```python
from build123d import *

# Parameters (mm, degrees)
ESBO_O1_R                = 1.5
RESSALTO_EXTRUS_O1_DEPTH = 2
ESBO_O2_R                = 1.5
RESSALTO_EXTRUS_O2_DEPTH = 1
ESBO_O4_R                = 2.5
ESBO_O4_R_2              = 1.5
RESSALTO_EXTRUS_O3_DEPTH = 2
ESBO_O5_R                = 1.5
RESSALTO_EXTRUS_O4_DEPTH = 2
ESBO_O6_R                = 1.648621548
RESSALTO_EXTRUS_O5_DEPTH = 1
ESBO_O7_W                = 11.938868243
ESBO_O7_H                = 15.738508052
CORTE_EXTRUS_O1_DEPTH    = 6
RESSALTO_EXTRUS_O6_START = -2
ESBO_O8_R                = 2.148621548
RESSALTO_EXTRUS_O6_DEPTH = 0.5
RESSALTO_EXTRUS_O7_START = -2.5
ESBO_O9_R                = 2.148621548
RESSALTO_EXTRUS_O7_DEPTH = 0.5
RESSALTO_EXTRUS_O8_START = -2.5
ESBO_O10_R               = 2
RESSALTO_EXTRUS_O8_DEPTH = 0.5
RESSALTO_EXTRUS_O9_START = -2
ESBO_O11_R               = 2
RESSALTO_EXTRUS_O9_DEPTH = 0.5


with BuildPart() as part:
    # Esboço1 → Ressalto-extrusão1 (new body)
    with BuildSketch(Plane.XY):
        with BuildLine():
            Line((-1.198777863, 9.438372785), (-2.475695902, 0.347749621))
            ThreePointArc((-2.475695902, 0.347749621), (-1.4263e-05, -2.5), (2.47569987, 0.347721373))
            Line((2.47569987, 0.347721373), (1.198866989, 9.438491296))
            ThreePointArc((1.198866989, 9.438491296), (-7.4142e-05, 11.839999998), (-1.198777863, 9.438372785))
        make_face()
        Circle(ESBO_O1_R, mode=Mode.SUBTRACT)
    extrude(amount=RESSALTO_EXTRUS_O1_DEPTH)

    # Esboço2 → Ressalto-extrusão2 (add)
    with BuildSketch(Plane.XY.offset(2)):
        with Locations(Location((0, 10.34, 0), (0, 0, 216.947631019))):
            Circle(ESBO_O2_R)
    extrude(amount=RESSALTO_EXTRUS_O2_DEPTH)

    # Espelhar1: part across plane


with BuildPart() as part_1:
    add(part.part)
    add(part.part.mirror(Plane(origin=(0, 10.34, 3), x_dir=(1, 0, 0), z_dir=(0, 0, 1))))

    # Esboço4 → Ressalto-extrusão3 (add)
    with BuildSketch(Plane.XY.offset(6)):
        with Locations(Location((0, 0, 0), (0, 0, 172.004238293))):
            Circle(ESBO_O4_R)
        Circle(ESBO_O4_R_2, mode=Mode.SUBTRACT)
    extrude(amount=RESSALTO_EXTRUS_O3_DEPTH)

    # Esboço5 → Ressalto-extrusão4 (add)
    with BuildSketch(Plane.XY.offset(8)):
        with BuildLine():
            Line((-6.643819561, 6.810437698), (-2.18535321, -1.21417929))
            ThreePointArc((-2.18535321, -1.21417929), (1.470887432, -2.021506904), (1.827663155, 1.705768857))
            Line((1.827663155, 1.705768857), (-4.435920088, 8.416947961))
            ThreePointArc((-4.435920088, 8.416947961), (-7.053565106, 9.69403249), (-6.643819561, 6.810437698))
        make_face()
        Circle(ESBO_O5_R, mode=Mode.SUBTRACT)
    extrude(amount=RESSALTO_EXTRUS_O4_DEPTH)

    # Esboço6 → Ressalto-extrusão5 (add)
    with BuildSketch(Plane.XY.offset(10)):
        with Locations(Location((-6.08359042, 8.360952554, 0), (0, 0, 250.134292883))):
            Circle(ESBO_O6_R)
    extrude(amount=RESSALTO_EXTRUS_O5_DEPTH)

    # Espelhar3: part across plane


with BuildPart() as part_2:
    add(part_1.part)
    add(part_1.part.mirror(Plane(origin=(-6.08359042, 8.360952554, 11), x_dir=(1, 0, 0), z_dir=(0, 0, 1))))

    # Esboço7 → Corte-extrusão1 (cut)
    with BuildSketch(Plane.XY.offset(22)):
        with Locations((-0.266328734, 4.470018957)):
            Rectangle(ESBO_O7_W, ESBO_O7_H)
    extrude(amount=-CORTE_EXTRUS_O1_DEPTH, mode=Mode.SUBTRACT)

    # Esboço8 → Ressalto-extrusão6 (add)
    with BuildSketch(Plane.XY.offset(14).offset(RESSALTO_EXTRUS_O6_START)):
        with Locations((-6.08359042, 8.360952554)):
            Circle(ESBO_O8_R)
    extrude(amount=-RESSALTO_EXTRUS_O6_DEPTH)

    # Esboço9 → Ressalto-extrusão7 (add)
    with BuildSketch(Plane(origin=(0, 0, 8), x_dir=(-1, 0, 0), z_dir=(0, 0, -1)).offset(RESSALTO_EXTRUS_O7_START)):
        with Locations(Location((6.08359042, 8.360952554, 0), (0, 0, 180))):
            Circle(ESBO_O9_R)
    extrude(amount=RESSALTO_EXTRUS_O7_DEPTH)

    # Esboço10 → Ressalto-extrusão8 (add)
    with BuildSketch(Plane(origin=(0, 0, 0), x_dir=(-1, 0, 0), z_dir=(0, 0, -1)).offset(RESSALTO_EXTRUS_O8_START)):
        with Locations(Location((0, 10.34, 0), (0, 0, 229.937782743))):
            Circle(ESBO_O10_R)
    extrude(amount=RESSALTO_EXTRUS_O8_DEPTH)

    # Esboço11 → Ressalto-extrusão9 (add)
    with BuildSketch(Plane.XY.offset(6).offset(RESSALTO_EXTRUS_O9_START)):
        with Locations(Location((0, 10.34, 0), (0, 0, 229.941078536))):
            Circle(ESBO_O11_R)
    extrude(amount=-RESSALTO_EXTRUS_O9_DEPTH)


solid = part_2.part
```
For this review, take the finished solid that the model builds, in its own axes (mm). A direction names the side the tool comes from. Round coordinates to 2 decimals unless told otherwise and drop trailing zeros. Loops run counter-clockwise (first coordinate to the right, second up) from the corner with the lowest first, then second, coordinate; pieces in that order, holes last.
Q1. Mouldability with a two-part tool opening along Z and no side actions: class faces 1 (the face through (-7, 10, 12)), 2 (the face through (-4, 5, 8)), 3 (the face through (-7.013, 9.723, 13.014)) as +Z half, -Z half, draft (parallel to the pull), parting line (faces both ways), or undercut.
Result sheet:
face 1: +Z half
face 2: undercut
face 3: draft
Q2. To check wall thickness, follow line 1 along Z through (x, y) = (1, 11.75); line 2 along Z through (x, y) = (0.75, 1.5); line 3 along Z through (x, y) = (-4.5, 9.5). State the ranges of each line that lie inside material, in increasing order.
Result sheet:
line 1: z = 2 to 2.5, 3.5 to 4
line 2: z = 0 to 2, 4 to 10, 12 to 16
line 3: z = 10 to 10.5, 11.5 to 12
Q3. Add section A-A on y = 4.5. Write out the cut boundary in (x, z), plus the area to 3 significant figures.
Result sheet:
outline: (-5.36, 8) - (-0.78, 8) - (-0.78, 10) - (-5.36, 10) - close; (-5.36, 12) - (-0.78, 12) - (-0.78, 14) - (-5.36, 14) - close; (-1.89, 0) - (1.89, 0) - (1.89, 2) - (-1.89, 2) - close; (-1.89, 4) - (1.89, 4) - (1.89, 6) - (-1.89, 6) - close
area: 33.5 mm2
Q4. Insertion check: pin 1 Ø1 at (x, y) = (-3, 1.5) entering from +Z; pin 2 Ø4 at (y, z) = (6.5, 10.5) entering from +X; pin 3 Ø4.5 at (x, y) = (-6.5, 8.5) entering from -Z; pin 4 Ø5 at (x, y) = (0, 0) entering from +Z. Each pin has a flat end and moves straight along its axis. Give the tip position at first contact, or say it passes through.
Result sheet:
pin 1: stops at z = 14
pin 2: stops at x = -0.84
pin 3: stops at z = 8
pin 4: stops at z = 16
Q5. Machinability: for faces 4 (the face through (-1.828, 4.957, 0.986)), 5 (the face through (-1.5, 0.07, 14.03)), 6 (the face through (0.05, 11.84, 5.01)), 7 (the face through (1, 9, 3.5)), 8 (the face through (-7.013, 9.723, 9.014)), which of the approach directions +Z, -Z, +X, -X, +Y, -Y give a long, thin tool a straight path to every point of the face, cutting with its end or side? Answer none if there is none.
Result sheet:
face 4: -Z, -X
face 5: +Z, -Z
face 6: +Z
face 7: none
face 8: -Z
Q6. Add section D-D on y = -0.5. Write out the cut boundary in (x, z).
Result sheet:
outline: (-2.58, 8) - (-2.45, 8) - (-2.45, 4) - (-1.41, 4) - (-1.41, 10) - (-2.58, 10) - close; (-2.58, 12) - (-1.41, 12) - (-1.41, 16) - (-2.45, 16) - (-2.45, 14) - (-2.58, 14) - close; (-2.45, 0) - (-1.41, 0) - (-1.41, 2) - (-2.45, 2) - close; (1.41, 0) - (2.45, 0) - (2.45, 2) - (1.41, 2) - close; (1.41, 4) - (2.45, 4) - (2.45, 10) - (1.41, 10) - close; (1.41, 12) - (2.45, 12) - (2.45, 16) - (1.41, 16) - close
Q7. Add section B-B on z = 13. Write out the cut boundary in (x, y), plus the area to 3 significant figures.
Result sheet:
outline: (-6.64, 6.81) - (-2.19, -1.21) arc R2.5 ccw (long way) to (1.83, 1.71) - (-4.44, 8.42) arc R1.65 ccw (long way) to start; hole circle Ø3 at (0, 0)
area: 46.5 mm2
Q8. Add section C-C on x = -1.75. Write out the cut boundary in (y, z), plus the area to 3 significant figures.
Result sheet:
outline: (-1.79, 0) - (5.51, 0) - (5.51, 2) - (-1.79, 2) - close; (-1.79, 4) - (5.51, 4) - (5.51, 6) - (1.79, 6) - (1.79, 8) - (5.54, 8) - (5.54, 10) - (-1.79, 10) - close; (-1.79, 12) - (5.54, 12) - (5.54, 14) - (1.79, 14) - (1.79, 16) - (-1.79, 16) - close; (9.37, 2) - (11.31, 2) - (11.31, 2.5) - (9.37, 2.5) - close; (9.37, 3.5) - (11.31, 3.5) - (11.31, 4) - (9.37, 4) - close
area: 74.7 mm2
